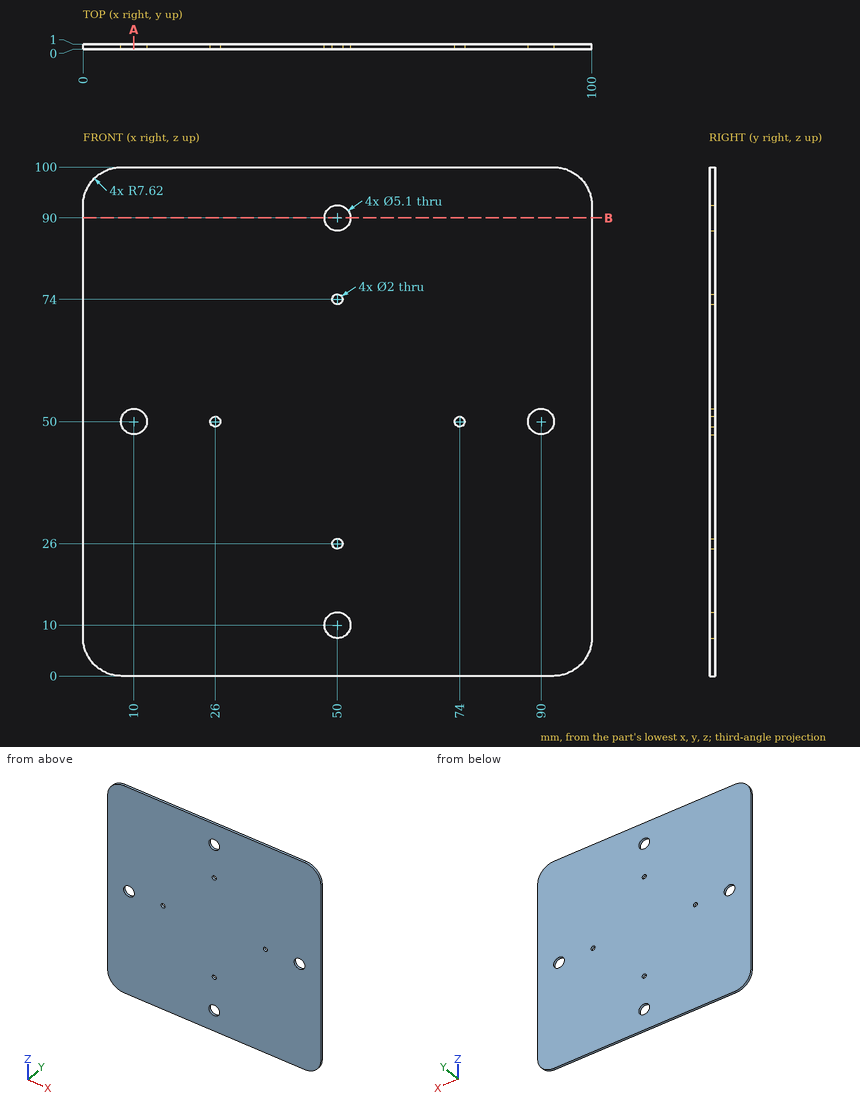
Input: dimensioned drawing with shaded views. Units: mm. Origin: part minimum x, y, z. Give positions to 0.01 mm unless a question says otherwise; leave off trailing zeros. Write each loop counter-clockwise with the first axis right and the second up, starting at its lowest first coordinate (ties: lowest second). Pieces come first, ordered by that corner, then holes. Notation, with made-up numbers: (27, -13.75) - (57, -13.75) arc R25 ccw to (57, 6.25) - close; hole circle Ø1 at (78, 71.5). An arc over 180 degrees is marked (long way). Write item = value, one per line. Start each with the question number.
1) Cut plane A-A (x = 10). Return loops of the section in (y, z).
2) Cut plane B-B (z = 90). Return loops of the section in (x, y), and give its area (3 significant figures).
3) Material intervals for L1, parallel to X at y = 0.7, z = 50; L2, parallel to X at y = 0.75, z = 10, sorted ascending. Write a range as [from, to].
4) Pin query (flat end, axial travel): pin 1 (1.6 mm diameter, centred on x = 26, z = 50, fed in from -Y). Return the tip coordinate at first contact, or that it passes through.
Answers follow:
q1.outline = (0, 0) - (1, 0) - (1, 47.45) - (0, 47.45) - close; (0, 52.55) - (1, 52.55) - (1, 100) - (0, 100) - close
q2.outline = (0, 0) - (47.45, 0) - (47.45, 1) - (0, 1) - close; (52.55, 0) - (100, 0) - (100, 1) - (52.55, 1) - close
q2.area = 94.9 mm^2
q3.L1 = [0, 7.45], [12.55, 25], [27, 73], [75, 87.45], [92.55, 100]
q3.L2 = [0, 47.45], [52.55, 100]
q4.pin_1 = through
